Autodesk Inventor part; units mm, degrees
ref_plane "YZ Plane" through (0, 0, 0) normal (1, 0, 0) x (0, 1, 0)
ref_plane "XZ Plane" through (0, 0, 0) normal (0, 1, 0) x (-1, 0, 0)
ref_plane "XY Plane" through (0, 0, 0) normal (0, 0, 1) x (1, 0, 0)
sketch "Náčrt1" plane through (0, 0, 0) normal (0, 1, 0) x (-1, 0, 0)
  line L0 (-49.75, 49.75) -> (49.75, 49.75)
  line L1 (49.75, 49.75) -> (49.75, -49.75)
  line L2 (49.75, -49.75) -> (-49.75, -49.75)
  line L3 (-49.75, -49.75) -> (-49.75, 49.75)
  line L4 (-49.75, 49.75) -> (49.75, -49.75) construction
  line L5 (49.75, 49.75) -> (-49.75, -49.75) construction
  line L6 (-19.75, 49.75) -> (-19.75, 23.75)
  line L7 (-19.75, 23.75) -> (-49.75, 23.75)
  line L8 (-49.75, -23.75) -> (-19.75, -23.75)
  line L9 (-19.75, -23.75) -> (-19.75, -49.75)
  circle A0 centre (-24.4375, -18.75) radius 1.75
  circle A1 centre (-24.4375, 18.75) radius 1.75
  line L10 (-39.25, 23.75) -> (-39.25, -23.75)
  circle A2 centre (-12.25, -42.25) radius 1.75
  circle A3 centre (39.7631, -20) radius 1.75
  circle A4 centre (39.7631, 20) radius 1.75
  circle A5 centre (-12.25, 42.25) radius 1.75
  circle A6 centre (41.75, 40.6105) radius 5
  circle A7 centre (41.75, -40.6105) radius 5
  line L11 (41.75, 40.6105) -> (41.75, 49.75) construction
  line L12 (41.75, -40.6105) -> (41.75, -49.75) construction
  circle A8 centre (-35.375, 0) radius 5
  line L13 (-35.375, 5) -> (-39.25, 5)
  line L14 (-35.375, -5) -> (-39.25, -5)
  line L15 (39.7631, 20) -> (39.7631, 0) construction
  line L16 (39.7631, 0) -> (39.7631, -20) construction
  point P0 (0, 0)
  point P1 (-34.75, 23.75)
  dimension "d0" = 99.5
  dimension "d1" = 99.5
  dimension "d2" = 30
  dimension "d3" = 26
  dimension "d4" = 10.5
  dimension "d5" = 3.5
  dimension "d7" = 7.5
  dimension "d8" = 7.5
  dimension "d9" = 5
  dimension "d10" = 5
  dimension "d11" = 10.3125
  dimension "d12" = 7.5
  dimension "d13" = 9.9869
  dimension "d26" = 81.221
  dimension "d27" = 10
  dimension "d28" = 8
  dimension "d29" = 10
  dimension "d30" = 3.875
  dimension "d31" = 40
extrude "Vysunutí1" add sketch "Náčrt1" along normal blind 5 contours L0 L1 L2 L9 L8 L10 L14 A8 L13 L7 L6 | A0 | A1 | A2 | A3 | A4 | A5
sketch "Náčrt2" plane through (-49.75, 0, 49.75) normal (0, 0, 1) x (1, 0, 0)
  line L0 (0, 0) -> (69.5, 0)
  line L1 (0, 0) -> (1.3397, 5)
  line L2 (0, 5) -> (69.5, 5)
  line L3 (0, 0) -> (0, 5)
  line L4 (0, 5) -> (0, 0)
  point P0 (49.75, 0)
  dimension "d16" = 75
extrude "Vysunutí2" cut sketch "Náčrt2" against normal through all
hole "Díra1" at (24.4375, 0, 18.75) at (24.4375, 0, -18.75) at (12.25, 0, -42.25) at (-39.7631, 0, -20) at (-39.7631, 0, 20) at (12.25, 0, 42.25) direction (0, 1, 0) diameter 3.5 end through all countersink diameter 7.5 countersink angle 90
properties part number "new_plech"
Verification items for the finished model (mm, model axes). A direction names the side the tool comes from. Give positions to 0.01 mm unless a question says otherwise; leave off trailing zeros. Loops run counter-clockwise (first coordinate to the right, second up) from the corner with the lowest first, then second, coordinate; pieces in that order, holes last.
1) Draft check along X on faces 1 (the cylindrical face through (-37.78, 2.46, -37.57)), 2 (the flat face through (19.75, 2, -37)), 3 (the flat face through (-5, 0, 1)). Enter one of: pulls with the +X half, pulls with the -X half, needs draft (parallel to the pull), parting line crosses it, or undercut.
2) Sectioned sample at B-B, the plane x = 32.5. Enter the section's corners in (y, z), then the cut area to 3 significant figures.
3) Depth check by flat-ended pin: pin 1 Ø1.9 at (x, y) = (37.5, 1.5) entering from -Z; pin 2 Ø4.5 at (x, z) = (24.44, 18.75) entering from -Y; pin 3 Ø1.2 at (x, y) = (38, 2) entering from +Z. Enter the tip coordinate at first touch or a pass-through.
4) Thickness scan on line 1 along Z through (x, y) = (12.25, 3.4); line 2 along X through (y, z) = (3.1, -20); line 3 along X through (y, z) = (2.7, 18.75). Record the ranges inside material, lowest first.
5) Sectioned sample at C-C, the plane z = 42.25. Enter the section's corners in (x, y).
6) Set-up check for faces 4 (the flat face through (37, 2, -5)), 5 (the flat face through (29, 2, 23.75)), 6 (the cylindrical face through (11.724, 3.521, 40.581)), 7 (the flat face through (30, 2, -23.75)): record each of +Z, -Z, +X, -X, +Y, -Y from which the full face is reachable in a straight line by a thin tool's end or side.
7) Sectioned sample at D-D, the plane z = 25. Enter the section's corners in (x, y).
8) Sectioned sample at A-A, the plane y = 1.05. Count the separate pieces of the cut face and the enclosed holes in it, then the cut area to 3 significant figures.
Answers:
1. face 1: undercut
1. face 2: pulls with the +X half
1. face 3: needs draft
2. outline: (0, -23.75) - (5, -23.75) - (5, -4.09) - (0, -4.09) - close; (0, 4.09) - (5, 4.09) - (5, 23.75) - (0, 23.75) - close
2. area: 197 mm2
3. pin 1: stops at z = -23.75
3. pin 2: stops at y = 1.5
3. pin 3: stops at z = 23.75
4. line 1: z = -49.75 to -44, -40.5 to 40.5, 44 to 49.75
4. line 2: x = -48.92 to -41.51, -38.01 to 23.21, 25.66 to 39.25
4. line 3: x = -49.03 to -40.99, -38.54 to 22.69, 26.19 to 39.25
5. outline: (-49.75, 0) - (-46.47, 0) - (-46.47, 5) - (-48.41, 5) - close; (-37.03, 0) - (8.5, 0) - (10.5, 2) - (10.5, 5) - (-37.03, 5) - close; (14, 2) - (16, 0) - (19.75, 0) - (19.75, 5) - (14, 5) - close
6. face 4: +X, +Y, -Y
6. face 5: +Z, +X, +Y, -Y
6. face 6: +Y, -Y
6. face 7: -Z, +X, +Y, -Y
7. outline: (-49.75, 0) - (19.75, 0) - (19.75, 5) - (-48.41, 5) - close
8. separate pieces: 1
8. enclosed holes: 8
8. area: 7,440 mm2
